```python
from build123d import *

# Parameters (mm, degrees)
BOSS_EXTRUDE1_DEPTH     = 50.8
SKETCH2_R               = 2.032
CUT_EXTRUDE1_DEPTH      = 12.43
CUT_EXTRUDE1_DEPTH_BACK = 7.35
CUT_EXTRUDE2_START      = -3.175
SKETCH3_R               = 3.81
CUT_EXTRUDE2_DEPTH      = 3.175


with BuildPart() as part:
    # Sketch1 → Boss-Extrude1 (new body)
    with BuildSketch(Plane(origin=(0, 0, 0), x_dir=(1, 0, 0), z_dir=(0, 1, 0))):
        with BuildLine():
            ThreePointArc((6.35, -18.272118104), (17.78, 0), (6.35, 18.272118104))
            Line((6.35, 18.272118104), (6.35, 25.4))
            Line((6.35, 25.4), (6.35, 31.75))
            Line((6.35, 31.75), (0, 31.75))
            Line((0, 31.75), (0, 13.73715036))
            ThreePointArc((0, 13.73715036), (11.43, 0), (0, -13.73715036))
            Line((0, -13.73715036), (0, -31.75))
            Line((0, -31.75), (6.35, -31.75))
            Line((6.35, -31.75), (6.35, -25.4))
            Line((6.35, -25.4), (6.35, -18.272118104))
        make_face()
    extrude(amount=BOSS_EXTRUDE1_DEPTH)

    # Sketch2 → Cut-Extrude1 (cut, two sides)
    with BuildSketch(Plane(origin=(6.35, 0, 0), x_dir=(0, 0, -1), z_dir=(1, 0, 0))) as cut_extrude1_sk:
        with Locations((25.011059052, 38.1)):
            Circle(SKETCH2_R)
        with Locations((25.011059052, 12.7)):
            Circle(SKETCH2_R)
        with Locations((-25.011059052, 12.7)):
            Circle(SKETCH2_R)
        with Locations((-25.011059052, 38.1)):
            Circle(SKETCH2_R)
    extrude(amount=CUT_EXTRUDE1_DEPTH, mode=Mode.SUBTRACT)
    extrude(cut_extrude1_sk.sketch, amount=-CUT_EXTRUDE1_DEPTH_BACK, mode=Mode.SUBTRACT)

    # Sketch3 → Cut-Extrude2 (cut)
    with BuildSketch(Plane(origin=(6.35, 0, 0), x_dir=(0, 0, -1), z_dir=(1, 0, 0)).offset(CUT_EXTRUDE2_START)):
        with Locations((25.011059052, 38.1)):
            Circle(SKETCH3_R)
        with Locations((25.011059052, 12.7)):
            Circle(SKETCH3_R)
        with Locations((-25.011059052, 38.1)):
            Circle(SKETCH3_R)
        with Locations((-25.011059052, 12.7)):
            Circle(SKETCH3_R)
    extrude(amount=CUT_EXTRUDE2_DEPTH, mode=Mode.SUBTRACT)


solid = part.part
```
Design review of the part built by this model. Coordinates are the model's own, in mm. A direction names the side the tool comes from. Round coordinates to 2 decimals unless told otherwise and drop trailing zeros. Write each loop counter-clockwise with the first axis right and the second up, starting at its lowest first coordinate (ties: lowest second). Pieces come first, ordered by that corner, then holes.
Item 1: For probe 1 along Y at (x, z) = (3.5, 26); probe 2 along Y at (x, z) = (6, -24.5); probe 3 along X at (y, z) = (18.5, 20), list the stretches that pass through material, from the lowest coordinate up.
Item 2: We need section D-D on z = 15.5. Write out the cut boundary in (x, y).
Item 3: The part is to be moulded in two halves that separate along Y. For faces 4 (the cylindrical face through (4.74, 34.38, 25.84)), 5 (the flat face through (13, 0, 0)), 6 (the flat face through (6.35, 25, -25)), say which applies: +Y half, -Y half, draft (parallel to the pull), parting line (faces both ways), or undercut.
Item 4: We need section C-C on y = 3. Write out the cut boundary in (x, z), and give its area (3 significant figures).
Item 5: Clearance check with flat-ended pins moving along their axes: pin 1 Ø7 at (y, z) = (38.1, -25.01) entering from +X (3 decimals); pin 2 Ø9 at (y, z) = (12.7, 25.01) entering from +X; pin 3 Ø15 at (y, z) = (21.5, -23) entering from +X. State where each tip first meets the part, or that it passes through.
Item 6: We need section B-B on x = 10. Write out the cut boundary in (y, z).
Item 7: For faces 1 (the flat face through (3.175, 36, -27)), 2 (the flat face through (0, 25, -23)), 3 (the flat face through (6.35, 25, 25)), list the 3-axis set-ups (+Z, -Z, +X, -X, +Y, -Y) from which the entire face can be reached by the end or side of a thin tool; tool diameter is ignored.
Item 8: We need section A-A on y = 38.1. Write out the cut boundary in (x, z) (3 decimals).
Returned:
1. probe 1: y = 0 to 9.02, 16.38 to 34.42, 41.78 to 50.8
1. probe 2: y = 0 to 8.92, 16.48 to 34.32, 41.88 to 50.8
1. probe 3: x = 0 to 6.35
2. outline: (0, 0) - (10.6, 0) - (10.6, 50.8) - (0, 50.8) - close
3. face 4: undercut
3. face 5: -Y half
3. face 6: draft
4. outline: (0, -31.75) - (6.35, -31.75) - (6.35, -18.27) arc R20.32 ccw to (6.35, 18.27) - (6.35, 31.75) - (0, 31.75) - (0, 13.74) arc R13.97 cw to (0, -13.74) - close
4. area: 466 mm2
5. pin 1: stops at x = 3.175
5. pin 2: stops at x = 6.35
5. pin 3: stops at x = 10.6
6. outline: (0, -15.99) - (50.8, -15.99) - (50.8, -6.16) - (0, -6.16) - close; (0, 6.16) - (50.8, 6.16) - (50.8, 15.99) - (0, 15.99) - close
7. face 1: +X
7. face 2: +Z, -Z, -X, +Y, -Y
7. face 3: +Z, +X, +Y, -Y
8. outline: (0, -31.75) - (6.35, -31.75) - (6.35, -28.821) - (3.175, -28.821) - (3.175, -27.043) - (0, -27.043) - close; (0, -22.979) - (3.175, -22.979) - (3.175, -21.201) - (6.35, -21.201) - (6.35, -18.272) arc R20.32 ccw to (6.35, 18.272) - (6.35, 21.201) - (3.175, 21.201) - (3.175, 22.979) - (0, 22.979) - (0, 13.737) arc R13.97 cw to (0, -13.737) - close; (0, 27.043) - (3.175, 27.043) - (3.175, 28.821) - (6.35, 28.821) - (6.35, 31.75) - (0, 31.75) - close
